```python
from build123d import *

# Parameters (mm, degrees)
F1_DEPTH        = 35
F3_DEPTH        = 17
F2_W            = 2.4522083601
F2_H            = 10
F2_W_2          = 2.5477916399
F2_W_3          = 32
F4_DEPTH        = 28.001
F5_W            = 2
F5_H            = 10
F6_DEPTH        = 14
F7_R            = 3
F8_DEPTH        = 40.001
F10_D           = 4.4
F10_CBORE_D     = 8.25
F10_CBORE_DEPTH = 4
F11_R           = 3.5
F11_R_2         = 2.2
F12_DEPTH       = 1.6


with BuildPart() as f1:
    # F0 (on Top) → F1 (new body)
    with BuildSketch(Plane.XY):
        Polygon((-34, 14), (0, 14), (0, 28), (-29, 28), (-40, 17), (-40, 7), (-37.4522083601, 0), (-32, 0), (-32, 2.5), (-34, 2.5), align=None)
    extrude(amount=-F1_DEPTH)

    # F2 (on face) → F3 (cut)
    with BuildSketch(Plane.XZ):
        with BuildLine():
            Line((0, 0), (-32, 0))
            Line((-32, 0), (-32, -9))
            ThreePointArc((-32, -9), (-30.5811388301, -9.7434164903), (-29, -10))
            Line((-29, -10), (0, -10))
            Line((0, -10), (0, 0))
        make_face()
        with BuildLine():
            Line((-32, 0), (-34, 0))
            Line((-34, 0), (-34, -5))
            ThreePointArc((-34, -5), (-33.472135955, -7.2360679775), (-32, -9))
            Line((-32, -9), (-32, 0))
        make_face()
    extrude(amount=-F3_DEPTH, mode=Mode.SUBTRACT)

    # F2 (on face) → F4 (cut, through all)
    with BuildSketch(Plane.XZ):
        with Locations((-36.2261041801, -30)):
            Rectangle(F2_W, F2_H)
        with Locations((-38.7261041801, -30)):
            Rectangle(F2_W_2, F2_H)
        with Locations((-16, -30)):
            Rectangle(F2_W_3, F2_H)
    extrude(amount=-F4_DEPTH, mode=Mode.SUBTRACT)

    # F5 (on face) → F6 (cut, through all)
    with BuildSketch(Plane(origin=(0, 28, 0), x_dir=(-1, 0, 0), z_dir=(0, 1, 0))):
        with Locations((33, -30)):
            Rectangle(F5_W, F5_H)
    extrude(amount=-F6_DEPTH, mode=Mode.SUBTRACT)

    # F7 (on face) → F8 (cut, through all)
    with BuildSketch(Plane.YZ):
        Polygon((23, -35), (23, -25), (14, -25), (14, -33), (14, -35), align=None)
        Polygon((14, -35), (14, -33), (12.8452994616, -35), align=None)
        with Locations((7, -19)):
            Circle(F7_R)
        Polygon((1.1547005384, -35), (0, -33), (0, -35), align=None)
    extrude(amount=-F8_DEPTH, mode=Mode.SUBTRACT)

    # F10 (through all)
    with Locations(Plane(origin=(0, 0, -25), x_dir=(1, 0, 0), z_dir=(0, 0, -1))):
        with Locations((-25.5, -22), (-7.5, -22)):
            CounterBoreHole(F10_D / 2, F10_CBORE_D / 2, F10_CBORE_DEPTH)

    # F11 (on face) → F12 (cut)
    with BuildSketch(Plane.XY):
        with Locations((-25.5, 22)):
            Circle(F11_R)
        with Locations((-25.5, 22)):
            Circle(F11_R_2, mode=Mode.SUBTRACT)
        with Locations((-7.5, 22)):
            Circle(F11_R)
        with Locations((-7.5, 22)):
            Circle(F11_R_2, mode=Mode.SUBTRACT)
    extrude(amount=-F12_DEPTH, mode=Mode.SUBTRACT)


solid = f1.part
```
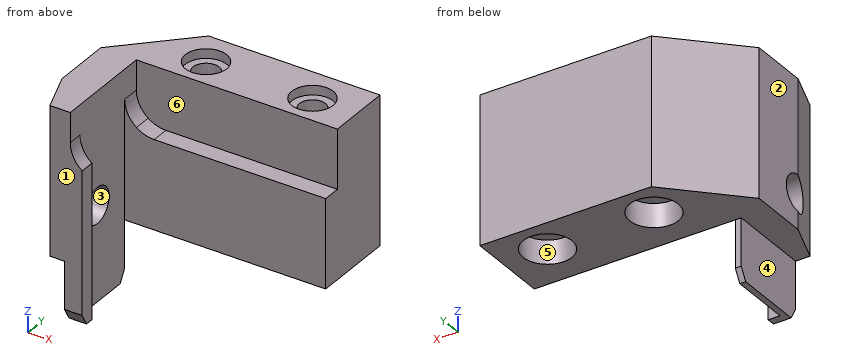
Geometry check sheet. Reference: the model listing, model coordinates, mm. Face numbers are marked on the shaded views. A direction names the side the tool comes from. Round coordinates to 2 decimals unless told otherwise and drop trailing zeros. Loops run counter-clockwise (first coordinate to the right, second up) from the corner with the lowest first, then second, coordinate; pieces in that order, holes last. Notation, with made-up numbers: M -11,37.5 L 4,37.5 A16 cw 4,61.5 Z; hole C 30.5,88 d1. An arc over 180 degrees is marked long. Return JSON: item names as keys, results as strings. Group by question number.
(1) Section check D-D, the plane z = -19. Enter the section's corners in (x, y), and give its area (3 significant figures).
(2) Go/stop test with flat-tipped pins: pin 1 (0.8 mm diameter, centred on x = -34.5, z = -28, fed in from +Y); pin 2 (5 mm diameter, centred on x = -25.5, y = 22, fed in from -Z); pin 3 (5 mm diameter, centred on y = 19, z = -27, fed in from -X); pin 4 (1.5 mm diameter, centred on y = 20.5, z = -15.5, fed in from +X). Record where each tip stops, or that it passes through.
(3) Set-up check for the marked faces 4, 5 and 6: record each of +Z, -Z, +X, -X, +Y, -Y from which the full face is reachable in a straight line by a thin tool's end or side.
(4) Mould release check, pull along Y, two halves, no side actions. Record for the marked faces 1, 2 and 3: pulls with the +Y half, pulls with the -Y half, needs draft (parallel to the pull), parting line crosses it, or undercut.
(5) Section check B-B, the plane y = 22. Enter the section's corners in (x, z) (3 decimals).
(6) Section check C-C, the plane z = -23.5. Enter the section's corners in (x, y) (3 decimals).
(7) Scan lines: line 1 along X through (y, z) = (22, -23.2) (3 decimals); line 2 along Y through (x, z) = (-7.5, -16.5); line 3 along Y through (x, z) = (-25.5, -0.65). Record each from-to range of solid material in increasing order. Write a range as [from, to].
(8) Section check A-A, the plane x = -7.5. Enter the section's corners in (y, z) (3 decimals), and give its area (3 significant figures).
Data:
{
 "1": {"outline": "M -40,10 L -34,10 L -34,14 L 0,14 L 0,28 L -29,28 L -40,17 Z; M -38.91,4 L -37.45,0 L -32,0 L -32,2.5 L -34,2.5 L -34,4 Z; hole C -25.5,22 d4.4; hole C -7.5,22 d4.4", "area": "515 mm²"},
 "2": {"pin 1": "y = 14", "pin 2": "z = -21", "pin 3": "x = -39.5", "pin 4": "x = 0"},
 "3": {"face 4": "-Z, -X, +Y, -Y", "face 5": "-Z", "face 6": "+Z, +X, -Y"},
 "4": {"face 1": "pulls with the -Y half", "face 2": "needs draft", "face 3": "undercut"},
 "5": {"outline": "M -35,-25 L -29.625,-25 L -29.625,-21 L -27.7,-21 L -27.7,-1.6 L -29,-1.6 L -29,0 L -35,0 Z; M -23.3,-21 L -21.375,-21 L -21.375,-25 L -11.625,-25 L -11.625,-21 L -9.7,-21 L -9.7,-1.6 L -11,-1.6 L -11,0 L -22,0 L -22,-1.6 L -23.3,-1.6 Z; M -5.3,-21 L -3.375,-21 L -3.375,-25 L 0,-25 L 0,0 L -4,0 L -4,-1.6 L -5.3,-1.6 Z"},
 "6": {"outline": "M -40,7 L -37.452,0 L -32,0 L -32,2.5 L -34,2.5 L -34,14 L 0,14 L 0,28 L -29,28 L -40,17 Z; hole C -25.5,22 d8.25; hole C -7.5,22 d8.25"},
 "7": {"line 1": "[-35, -29.625], [-21.375, -11.625], [-3.375, 0]", "line 2": "[14, 19.8], [24.2, 28]", "line 3": "[17, 18.5], [25.5, 28]"},
 "8": {"outline": "M 14,-25 L 17.875,-25 L 17.875,-21 L 19.8,-21 L 19.8,-1.6 L 18.5,-1.6 L 18.5,0 L 17,0 L 17,-10 L 14,-10 Z; M 24.2,-21 L 26.125,-21 L 26.125,-25 L 28,-25 L 28,0 L 25.5,0 L 25.5,-1.6 L 24.2,-1.6 Z", "area": "190 mm²"}
}
